Read the model definition and answer for the solid it produces. Units are mm, in the model's axes. A direction names the side the tool comes from. Round coordinates to 2 decimals unless told otherwise and drop trailing zeros. Write each loop counter-clockwise with the first axis right and the second up, starting at its lowest first coordinate (ties: lowest second). Pieces come first, ordered by that corner, then holes. Notation, with made-up numbers: (21.25, 87) -> (59.25, 87) arc R5 cw to (59.25, 91) -> close; hole circle Ø2 at (51, 8). An arc over 180 degrees is marked (long way). Return JSON: item names as keys, results as strings. Group by question number.
(1) Given pin 1 (16 mm diameter, centred on x = 33.5, z = 20.5, fed in from +Y); pin 2 (11 mm diameter, centred on y = 0, z = 41, fed in from -X); pin 3 (7 mm diameter, centred on x = -35.1, z = 15, fed in from -Y); pin 4 (6 mm diameter, centred on x = 33, y = 13, fed in from -Z), each flat-ended and moving along its own axis, determine where each tip first touches the part or whether it passes through.
(2) A cutting plane is placed at B-B on z = 15. Give the vertices of the cut face in (x, y).
(3) A cutting plane is placed at D-D on y = 17. Give the vertices of the cut face in (x, z).
(4) Straight lines are drawn through the part: line 1 (Z direction, x = -35.1, y = -0.75); line 2 (Y direction, x = -29.5, z = 35); line 3 (Z direction, x = -29.5, y = -42.5). For each, find the intervals that lie inside material, in ascending order.
(5) A cutting plane is placed at A-A on y = 1.5. Give the vertices of the cut face in (x, z), then the cut area to 3 significant figures.
(6) For faces 1 (the flat face through (30, -5, 35)), 2 (the flat face through (20.1, 0, 26)), 3 (the flat face through (-30, 5, 35)), determine the directions among +Z, -Z, +X, -X, +Y, -Y from which every point of the face is accessible in a straight line to the end or side of a thin tool.
(7) The mould has two halves that part along Y. Classify faces 4 (the flat face through (-1, -50, 2)), 5 (the flat face through (-20.1, 0, 26)), 6 (the flat face through (40.1, 0, 35)), 7 (the flat face through (0, 20.1, 3)): released by +Y, released by -Y, zero draft, split by the parting line, or undercut.
(8) A cutting plane is placed at C-C on x = -35.1. Give the vertices of the cut face in (y, z).
```python
from build123d import *

# Parameters (mm, degrees)
SKETCH_W        = 100
SKETCH_H        = 100
PAD_DEPTH       = 5
SKETCH001_W     = 40.2
SKETCH001_H     = 40.2
POCKET_DEPTH    = 5
SKETCH002_W     = 20
SKETCH002_H     = 10
PAD001_DEPTH    = 60
SKETCH003_R     = 2.25
POCKET001_DEPTH = 10


with BuildPart() as part:
    # Sketch → Pad (new body)
    with BuildSketch(Plane.XY):
        Rectangle(SKETCH_W, SKETCH_H)
    extrude(amount=PAD_DEPTH)

    # Sketch001 (on DatumPlane) → Pocket (cut)
    with BuildSketch(Plane.XY.offset(5)):
        Rectangle(SKETCH001_W, SKETCH001_H)
    extrude(amount=-POCKET_DEPTH, mode=Mode.SUBTRACT)

    # Sketch002 (on DatumPlane) → Pad001 (join)
    with BuildSketch(Plane.XY.offset(5)):
        with Locations((-30.1, 0)):
            Rectangle(SKETCH002_W, SKETCH002_H)
        with Locations((30.1, 0)):
            Rectangle(SKETCH002_W, SKETCH002_H)
    extrude(amount=PAD001_DEPTH)

    # Sketch003 (on DatumPlane) → Pocket001 (cut)
    with BuildSketch(Plane.XZ.offset(5)):
        with Locations((-35.1, 15)):
            Circle(SKETCH003_R)
        with Locations((35.1, 15)):
            Circle(SKETCH003_R)
        with Locations((-35.1, 35)):
            Circle(SKETCH003_R)
        with Locations((-35.1, 55)):
            Circle(SKETCH003_R)
        with Locations((-35.1, 75)):
            Circle(SKETCH003_R)
        with Locations((35.1, 75)):
            Circle(SKETCH003_R)
        with Locations((35.1, 55)):
            Circle(SKETCH003_R)
        with Locations((35.1, 35)):
            Circle(SKETCH003_R)
    extrude(amount=-POCKET001_DEPTH, mode=Mode.SUBTRACT)


solid = part.part
```
Checks:
{
 "1": {"pin 1": "stops at y = 5", "pin 2": "stops at x = -40.1", "pin 3": "stops at y = -5", "pin 4": "stops at z = 0"},
 "2": {"outline": "(-40.1, -5) -> (-37.35, -5) -> (-37.35, 5) -> (-40.1, 5) -> close; (-32.85, -5) -> (-20.1, -5) -> (-20.1, 5) -> (-32.85, 5) -> close; (20.1, -5) -> (32.85, -5) -> (32.85, 5) -> (20.1, 5) -> close; (37.35, -5) -> (40.1, -5) -> (40.1, 5) -> (37.35, 5) -> close"},
 "3": {"outline": "(-50, 0) -> (-20.1, 0) -> (-20.1, 5) -> (-50, 5) -> close; (20.1, 0) -> (50, 0) -> (50, 5) -> (20.1, 5) -> close"},
 "4": {"line 1": "z = 0 to 12.75, 17.25 to 32.75, 37.25 to 52.75, 57.25 to 65", "line 2": "y = -5 to 5", "line 3": "z = 0 to 5"},
 "5": {"outline": "(-50, 0) -> (-20.1, 0) -> (-20.1, 65) -> (-40.1, 65) -> (-40.1, 5) -> (-50, 5) -> close; (20.1, 0) -> (50, 0) -> (50, 5) -> (40.1, 5) -> (40.1, 65) -> (20.1, 65) -> close; hole circle Ø4.5 at (-35.1, 15); hole circle Ø4.5 at (-35.1, 35); hole circle Ø4.5 at (-35.1, 55); hole circle Ø4.5 at (35.1, 15); hole circle Ø4.5 at (35.1, 35); hole circle Ø4.5 at (35.1, 55)", "area": "2,600 mm^2"},
 "6": {"face 1": "+Z, +X, -X, -Y", "face 2": "+Z, -Z", "face 3": "+Z, +X, -X, +Y"},
 "7": {"face 4": "released by -Y", "face 5": "undercut", "face 6": "zero draft", "face 7": "undercut"},
 "8": {"outline": "(-50, 0) -> (50, 0) -> (50, 5) -> (5, 5) -> (5, 12.75) -> (-5, 12.75) -> (-5, 5) -> (-50, 5) -> close; (-5, 17.25) -> (5, 17.25) -> (5, 32.75) -> (-5, 32.75) -> close; (-5, 37.25) -> (5, 37.25) -> (5, 52.75) -> (-5, 52.75) -> close; (-5, 57.25) -> (5, 57.25) -> (5, 65) -> (-5, 65) -> close"}
}
